Input: part model. Units: mm. Frame: model coordinates. A direction names the side the tool comes from. Round coordinates to 2 decimals unless told otherwise and drop trailing zeros. Loops run counter-clockwise (first coordinate to the right, second up) from the corner with the lowest first, then second, coordinate; pieces in that order, holes last. Notation, with made-up numbers: M 24.25,0 L 28.25,0 A27 cw 28.25,21 Z; hole C -7,49 d6. An arc over 180 degrees is marked long. Return JSON: item names as keys, results as strings. Group by question number.
1) Section A-A (y = 0). Output: boundary loops of the cut face in (x, z), plus the area to 4 significant figures.
2) Access query for faces 3 (the face through (0, -2, 0)), 4 (the face through (0, 0, -10.15)), 5 (the face through (1.3, -2, -1.15)). Directions: +Z, -Z, +X, -X, +Y, -Y. A direction counts if a zero-diameter tool reaches every point of the face in a straight line with its end or side. Return the directions, or none.
3) Section C-C (z = 8). Output: boundary loops of the cut face in (x, y).
4) Material intervals for line 1 (Z direction, x = -1.7, y = -2.2); line 2 (Z direction, x = 1.85, y = -0.85); line 3 (X direction, y = 1.9, z = -1.5), sorted ascending. Write a range as from..to.
5) Section D-D (z = -2). Output: boundary loops of the cut face in (x, y).
6) Contact query for flat-ended pins moving along their axis: P1, Ø2, axis at y = 0, z = -3, coming from the +X side; P2, Ø1.5, axis at y = 0.5, z = 1, coming from the +X side; P3, Ø2, axis at x = 1, z = 5.5, coming from the -Y side. Output: stop coordinate, or through.
7) Mould query, pull axis Y, two halves, no side actions, for faces 1 (the face through (-2.15, 0.09, -5.59)), 2 (the face through (0, 0, 13.5)). Classes: +Y half, -Y half, draft (parallel to the pull), parting line (faces both ways), or undercut.
Autodesk Inventor part; units mm, degrees
ref_plane "YZ Plane" through (0, 0, 0) normal (1, 0, 0) x (0, 1, 0)
ref_plane "XZ Plane" through (0, 0, 0) normal (0, 1, 0) x (-1, 0, 0)
ref_plane "XY Plane" through (0, 0, 0) normal (0, 0, 1) x (1, 0, 0)
sketch "스케치1" plane through (0, 0, 0) normal (0, 0, 1) x (1, 0, 0)
  circle A0 centre (0, 0) radius 1.75
  circle A1 centre (0, 0) radius 3
  circle A2 centre (0, 0) radius 2.15
  dimension "d0" = 3.5
  dimension "d1" = 6
  dimension "d2" = 4.3
extrude "돌출1" add sketch "스케치1" along normal blind 13.5 contours A0
extrude "돌출2" add sketch "스케치1" against normal blind 1.15 contours A0 | A1 | A2
extrude "돌출3" add sketch "스케치1" against normal blind 10.15 contours A0 | A2
chamfer "모따기1" distance 1 angle 45 1 edges at (-1.75, 0, 13.5)
properties part number "Audio_jac"
Returned:
{
 "1": {"outline": "M -3,-1.15 L -2.15,-1.15 L -2.15,-10.15 L 2.15,-10.15 L 2.15,-1.15 L 3,-1.15 L 3,0 L 1.75,0 L 1.75,12.5 L 0.75,13.5 L -0.75,13.5 L -1.75,12.5 L -1.75,0 L -3,0 Z", "area": "91.85 mm^2"},
 "2": {"face 3": "+Z", "face 4": "-Z, +X, -X, +Y, -Y", "face 5": "-Z"},
 "3": {"outline": "C 0,0 d3.5"},
 "4": {"line 1": "z = -1.15..0", "line 2": "z = -10.15..0", "line 3": "x = -1.01..1.01"},
 "5": {"outline": "C 0,0 d4.3"},
 "6": {"P1": "stops at x = 2.15", "P2": "stops at x = 1.75", "P3": "stops at y = -1.75"},
 "7": {"face 1": "parting line", "face 2": "draft"}
}
